Work out the finished part from the listing and answer in its coordinate system (mm). Face numbers are marked on the shaded views. Coordinates: 2 decimals unless noted, no trailing zeros. Order: outer loops, then holes, each group sorted by start corner. A loop starts at its lowest first (then second) coordinate and runs counter-clockwise, first axis right, second up. Notation, with made-up numbers: M 34,86.5 L 83,86.5 A29 ccw 83,111.5 Z; hole C 37,83.25 d3. An arc over 180 degrees is marked long. Write item = value, one per line. Start each with the question number.
Q1. Straight lines are drawn through the part: line 1 along Y through (x, z) = (-0.75, -2.25); line 2 along Z through (x, y) = (0, 24); line 3 along Z through (x, y) = (1, 17.5). For each, find the intervals that lie inside material, in ascending order.
Q2. Each of these flat-tipped pins is pushed along its axis until it touches: P1, Ø1.5, axis at x = 1, y = 33.5, coming from the +Z side; P2, Ø0.5, axis at x = 3, y = 31, coming from the -Z side; P3, Ø2.5, axis at y = 6, z = 2.5, coming from the -X side; P4, Ø2.5, axis at x = 0, z = 0, coming from the -Y side. Where does it stop, or does it pass through?
Q3. Find section D-D on y = 24. Give the vertices of the cut face in (x, z), and give its area (3 significant figures).
Q4. Find section B-B on z = 0. Give the vertices of the cut face in (x, y).
Q5. Find section C-C on z = -3.5. Give the vertices of the cut face in (x, y), and give its area (3 significant figures).
Q6. Find section A-A on x = 0. Give the vertices of the cut face in (y, z).
Q7. Determine the mould class of the marked faces 1, 2 and 3 for opening direction X: released by +X, released by -X, zero draft, split by the parting line, or undercut.
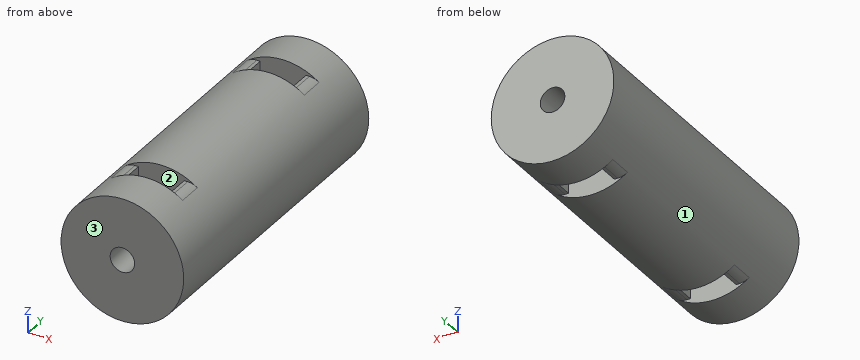
```python
from build123d import *

# Parameters (mm, degrees)
SKETCH1_R           = 7.5
SKETCH1_R_2         = 1.5
BOSS_EXTRUDE1_DEPTH = 38
SKETCH2_W           = 5.6
SKETCH2_H           = 17.764538462
CUT_EXTRUDE1_DEPTH  = 3
SKETCH3_W           = 5.6
SKETCH3_H           = 17.764538462
CUT_EXTRUDE2_DEPTH  = 3
SKETCH4_W           = 28.563856461
SKETCH4_H           = 7.504556993
SKETCH4_W_2         = 23.531731035
SKETCH4_H_2         = 6.282884924
CUT_EXTRUDE3_DEPTH  = 3
SKETCH5_W           = 28.563856461
SKETCH5_H           = 7.504556993
SKETCH5_W_2         = 23.531731035
SKETCH5_H_2         = 6.282884924
CUT_EXTRUDE4_DEPTH  = 3
FILLET1_R           = 2


with BuildPart() as part:
    # Sketch1 → Boss-Extrude1 (new body)
    with BuildSketch(Plane(origin=(0, 0, 0), x_dir=(1, 0, 0), z_dir=(0, 1, 0))):
        Circle(SKETCH1_R)
        Circle(SKETCH1_R_2, mode=Mode.SUBTRACT)
    extrude(amount=BOSS_EXTRUDE1_DEPTH)

    # Sketch2 → Cut-Extrude1 (cut)
    with BuildSketch(Plane(origin=(0, 33, 0), x_dir=(1, 0, 0), z_dir=(0, 1, 0))):
        Rectangle(SKETCH2_W, SKETCH2_H)
    extrude(amount=-CUT_EXTRUDE1_DEPTH, mode=Mode.SUBTRACT)

    # Sketch3 → Cut-Extrude2 (cut)
    with BuildSketch(Plane(origin=(0, 5, 0), x_dir=(-1, 0, 0), z_dir=(0, -1, 0))):
        Rectangle(SKETCH3_W, SKETCH3_H)
    extrude(amount=-CUT_EXTRUDE2_DEPTH, mode=Mode.SUBTRACT)

    # Sketch4 → Cut-Extrude3 (cut)
    with BuildSketch(Plane(origin=(0, 33, 0), x_dir=(1, 0, 0), z_dir=(0, 1, 0))):
        with Locations((0.852860298, 10.210008012)):
            Rectangle(SKETCH4_W, SKETCH4_H)
        with Locations((0.954666304, -9.599171977)):
            Rectangle(SKETCH4_W_2, SKETCH4_H_2)
    extrude(amount=-CUT_EXTRUDE3_DEPTH, mode=Mode.SUBTRACT)

    # Sketch5 → Cut-Extrude4 (cut)
    with BuildSketch(Plane(origin=(0, 5, 0), x_dir=(-1, 0, 0), z_dir=(0, -1, 0))):
        with Locations((-0.852860298, 10.210008012)):
            Rectangle(SKETCH5_W, SKETCH5_H)
        with Locations((-0.954666304, -9.599171977)):
            Rectangle(SKETCH5_W_2, SKETCH5_H_2)
    extrude(amount=-CUT_EXTRUDE4_DEPTH, mode=Mode.SUBTRACT)

    # Fillet1
    fillet1_edges = [part.edges().sort_by_distance(p)[0] for p in [
        (-3.814148596, 6.5, -6.457729515),
        (3.814148596, 6.5, -6.457729515),
        (3.814148596, 6.5, 6.457729515),
        (-3.814148596, 6.5, 6.457729515),
        (-3.814148596, 31.5, -6.457729515),
        (3.814148596, 31.5, -6.457729515),
        (3.814148596, 31.5, 6.457729515),
        (-3.814148596, 31.5, 6.457729515),
    ]]
    fillet(fillet1_edges, radius=FILLET1_R)


solid = part.part
```
Findings below:
q1.line_1 = 0 to 5, 8 to 30, 33 to 38
q1.line_2 = -7.5 to -1.5, 1.5 to 7.5
q1.line_3 = -7.43 to -1.12, 1.12 to 7.43
q2.P1 = 7.5
q2.P2 = -6.46
q2.P3 = -7.4
q2.P4 = through
q3.outline = C 0,0 d15; hole C 0,0 d3
q3.area = 170 mm^2
q4.outline = M -7.5,0 L -1.5,0 L -1.5,5 L -2.8,5 L -2.8,8 L -1.5,8 L -1.5,30 L -2.8,30 L -2.8,33 L -1.5,33 L -1.5,38 L -7.5,38 Z; M 1.5,0 L 7.5,0 L 7.5,38 L 1.5,38 L 1.5,33 L 2.8,33 L 2.8,30 L 1.5,30 L 1.5,8 L 2.8,8 L 2.8,5 L 1.5,5 Z
q5.outline = M -6.63,0 L 6.63,0 L 6.63,38 L -6.63,38 Z; hole M -2.8,5 L 2.8,5 L 2.8,8 L -2.8,8 Z; hole M -2.8,30 L 2.8,30 L 2.8,33 L -2.8,33 Z
q5.area = 471 mm^2
q6.outline = M 0,-7.5 L 5,-7.5 L 5,-1.5 L 0,-1.5 Z; M 0,1.5 L 5,1.5 L 5,7.5 L 0,7.5 Z; M 8,-7.5 L 30,-7.5 L 30,-1.5 L 8,-1.5 Z; M 8,1.5 L 30,1.5 L 30,7.5 L 8,7.5 Z; M 33,-7.5 L 38,-7.5 L 38,-1.5 L 33,-1.5 Z; M 33,1.5 L 38,1.5 L 38,7.5 L 33,7.5 Z
q7.face_1 = split by the parting line
q7.face_2 = undercut
q7.face_3 = zero draft
